```python
from build123d import *

# Parameters (mm, degrees)
F0_R     = 50
F1_DEPTH = 3
F2_DEPTH = 3
F4_DEPTH = 25


with BuildPart() as f1:
    # F0 (on Top) → F1 (new body)
    with BuildSketch(Plane.XY):
        Circle(F0_R)
        with BuildLine():
            Line((-16.798327, -18.869394), (-5, -7.071068))
            Line((-5, -7.071068), (-5, -39.68627))
            ThreePointArc((-5, -39.68627), (-16.930856, -36.240118), (-27.229775, -29.300842))
            Line((-27.229775, -29.300842), (-16.798327, -18.869394))
        make_face(mode=Mode.SUBTRACT)
        with BuildLine():
            Line((5, -39.68627), (5, -7.071068))
            Line((5, -7.071068), (15.141531, -17.212599))
            Line((15.141531, -17.212599), (27.229775, -29.300842))
            ThreePointArc((27.229775, -29.300842), (16.930856, -36.240118), (5, -39.68627))
        make_face(mode=Mode.SUBTRACT)
        with BuildLine():
            ThreePointArc((-33.668346, -21.597279), (-36.231596, 16.949083), (-5, 39.68627))
            Line((-5, 39.68627), (-5, 7.071068))
            Line((-5, 7.071068), (-23.869394, -11.798327))
            Line((-23.869394, -11.798327), (-33.668346, -21.597279))
        make_face(mode=Mode.SUBTRACT)
        with BuildLine():
            Line((11.400651, 0), (5, 6.400651))
            Line((5, 6.400651), (5, 39.68627))
            ThreePointArc((5, 39.68627), (36.333601, 16.729299), (33.404229, -22.003578))
            Line((33.404229, -22.003578), (21.87739, -10.476739))
            Line((21.87739, -10.476739), (11.400651, 0))
        make_face(mode=Mode.SUBTRACT)
    extrude(amount=F1_DEPTH)

    # F0 (on Top) → F2 (join)
    with BuildSketch(Plane.XY):
        Circle(F0_R)
        with BuildLine():
            Line((-16.798327, -18.869394), (-5, -7.071068))
            Line((-5, -7.071068), (-5, -39.68627))
            ThreePointArc((-5, -39.68627), (-16.930856, -36.240118), (-27.229775, -29.300842))
            Line((-27.229775, -29.300842), (-16.798327, -18.869394))
        make_face(mode=Mode.SUBTRACT)
        with BuildLine():
            Line((5, -39.68627), (5, -7.071068))
            Line((5, -7.071068), (15.141531, -17.212599))
            Line((15.141531, -17.212599), (27.229775, -29.300842))
            ThreePointArc((27.229775, -29.300842), (16.930856, -36.240118), (5, -39.68627))
        make_face(mode=Mode.SUBTRACT)
        with BuildLine():
            ThreePointArc((-33.668346, -21.597279), (-36.231596, 16.949083), (-5, 39.68627))
            Line((-5, 39.68627), (-5, 7.071068))
            Line((-5, 7.071068), (-23.869394, -11.798327))
            Line((-23.869394, -11.798327), (-33.668346, -21.597279))
        make_face(mode=Mode.SUBTRACT)
        with BuildLine():
            Line((11.400651, 0), (5, 6.400651))
            Line((5, 6.400651), (5, 39.68627))
            ThreePointArc((5, 39.68627), (36.333601, 16.729299), (33.404229, -22.003578))
            Line((33.404229, -22.003578), (21.87739, -10.476739))
            Line((21.87739, -10.476739), (11.400651, 0))
        make_face(mode=Mode.SUBTRACT)
    extrude(amount=F2_DEPTH)

    # F3 (on face) → F4 (cut)
    with BuildSketch(Plane.XY.offset(3)):
        with BuildLine():
            ThreePointArc((0, 42), (2.12132, 42.87868), (3, 45))
            ThreePointArc((3, 45), (-2.12132, 47.12132), (0, 42))
        make_face()
    extrude(amount=-F4_DEPTH, mode=Mode.SUBTRACT)


solid = f1.part
```
For this review, take the finished solid that the model builds, in its own axes (mm). A direction names the side the tool comes from. Round coordinates to 2 decimals unless told otherwise and drop trailing zeros. Write each loop counter-clockwise with the first axis right and the second up, starting at its lowest first coordinate (ties: lowest second). Pieces come first, ordered by that corner, then holes. Notation, with made-up numbers: (45, -11.75) -> (87, -11.75) arc R27 cw to (87, 7.25) -> close; hole circle Ø2 at (-16, -10.75). An arc over 180 degrees is marked (long way). Use one line per item in the form item = value.
1) Tool access review of faces 1 (the flat face through (-5, -23, 1)), 2 (the flat face through (-1, 1, 0)): name each direction out of +Z, -Z, +X, -X, +Y, -Y from which nothing blocks a thin tool from reaching the whole face with its end or side.
Found:
face_1 = +Z, -Z
face_2 = -Z, +X, -X, +Y, -Y
2) Clearance check with flat-ended pins moving along their axes: pin 1 (1.5 mm diameter, centred on y = 26, z = 1, fed in from -X); pin 2 (1.5 mm diameter, centred on x = 38, y = -26.5, fed in from -Z); pin 3 (1 mm diameter, centred on x = -9.5, z = 1.5, fed in from +Y); pin 4 (1.5 mm diameter, centred on x = 28.5, z = 1.5, fed in from +Y). State where each tip first meets the part, or that it passes through.
Found:
pin_1 = -43.16
pin_2 = 0
pin_3 = 49.18
pin_4 = 41.59
3) Take a section at B-B, the plane y = 9.5. Write out the cut boundary in (x, z), and give its area (3 significant figures).
Found:
outline = (-49.09, 0) -> (-38.86, 0) -> (-38.86, 3) -> (-49.09, 3) -> close; (-5, 0) -> (5, 0) -> (5, 3) -> (-5, 3) -> close; (38.86, 0) -> (49.09, 0) -> (49.09, 3) -> (38.86, 3) -> close
area = 91.4 mm2
4) Take a section at D-D, the plane y = -42.5. Write out the cut boundary in (x, z).
Found:
outline = (-26.34, 0) -> (26.34, 0) -> (26.34, 3) -> (-26.34, 3) -> close
5) Take a section at C-C, the plane x = 21. Write out the cut boundary in (y, z).
Found:
outline = (-45.38, 0) -> (-34.04, 0) -> (-34.04, 3) -> (-45.38, 3) -> close; (-23.07, 0) -> (-9.6, 0) -> (-9.6, 3) -> (-23.07, 3) -> close; (34.04, 0) -> (45.38, 0) -> (45.38, 3) -> (34.04, 3) -> close
6) To check wall thickness, follow L1, parallel to Y at x = 0, z = 2.2; L2, parallel to X at y = -17, z = 2.35; L3, parallel to Y at x = 22, z = 2.5. State the ranges of each line that lie inside material, in increasing order. Write a range as from..to.
Found:
L1 = -50..42, 48..50
L2 = -47.02..-36.21, -29.07..-14.93, -5..5, 14.93..28.4, 36.21..47.02
L3 = -44.9..-33.41, -24.07..-10.6, 33.41..44.9
7) Take a section at A-A, the plane z = 0.5. Write out the cut boundary in (x, y).
Found:
outline = circle Ø100 at (0, 0); hole (-33.67, -21.6) -> (-5, 7.07) -> (-5, 39.69) arc R40 ccw to start; hole (-27.23, -29.3) arc R40 ccw to (-5, -39.69) -> (-5, -7.07) -> close; hole (0, 42) arc R3 ccw to (3, 45) arc R3 ccw (long way) to start; hole (5, -39.69) arc R40 ccw to (27.23, -29.3) -> (5, -7.07) -> close; hole (5, 6.4) -> (33.4, -22) arc R40 ccw to (5, 39.69) -> close
8) Mouldability with a two-part tool opening along Y and no side actions: class faces 3 (the cylindrical face through (47.69, 15.02, 1.48)), 4 (the flat face through (19.4, -8, 1.5)), 5 (the flat face through (-1, 1, 3)) as +Y half, -Y half, draft (parallel to the pull), parting line (faces both ways), or undercut.
Found:
face_3 = parting line
face_4 = undercut
face_5 = draft
